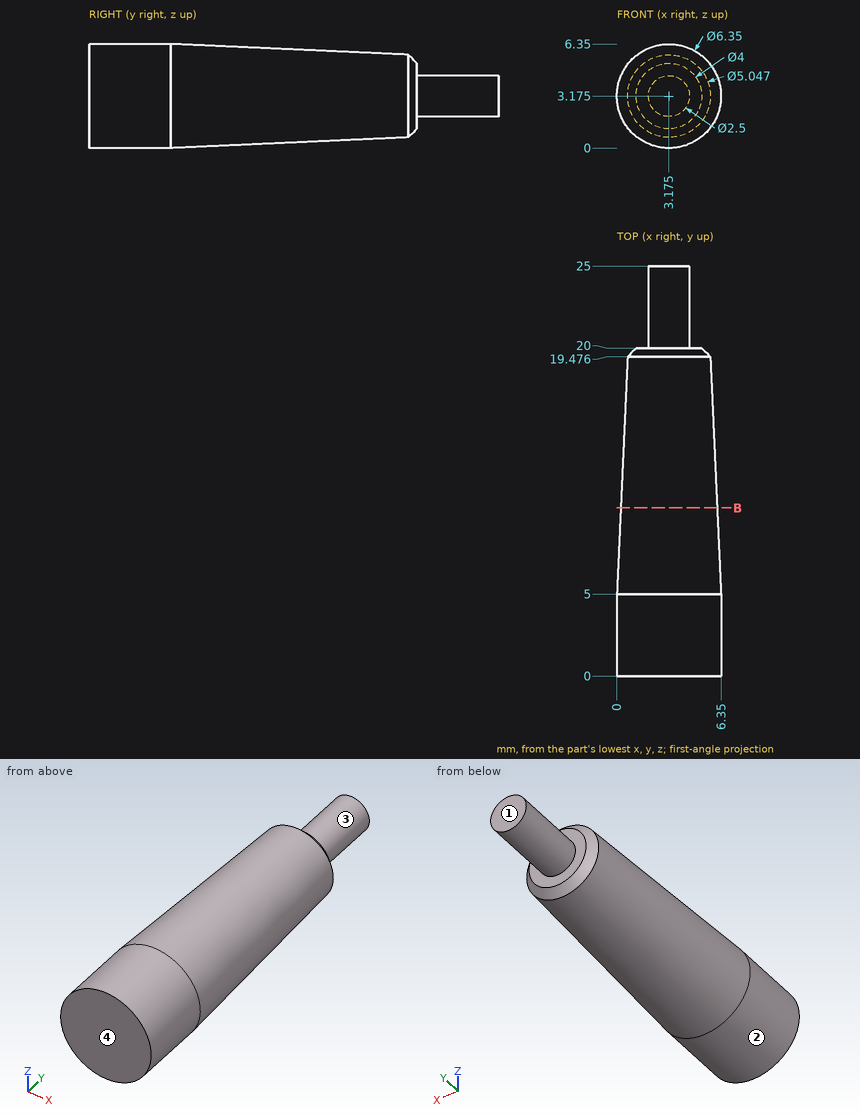
Source: three-view drawing plus pictorial views. Frame: mm from the lowest corner of the part. A direction names the side the tool comes from. Round coordinates to 2 decimals unless told otherwise and drop trailing zeros. Loops run counter-clockwise (first coordinate to the right, second up) from the corner with the lowest first, then second, coordinate; pieces in that order, holes last. Notation, with made-up numbers: M -27.75,-18.5 L 20.25,-18.5 A17 cw 20.25,-0.5 Z; hole C 43,39.25 d1. An arc over 180 degrees is marked long. Answer as CSV lines item,"result". Start each with the question number.
(1) Line query: line 1 (Y direction, x = 2.25, z = 1.5); line 2 (Z direction, x = 2, y = 6.75); line 3 (Z direction, x = 2.5, y = 16.75) (1 decimal). Output: solid intervals per line, ascending. Write a range as [from, to].
(2) First-contact query: pin 1 (3 mm diameter, centred on y = 4, z = 4.5, fed in from -X); pin 2 (2 mm diameter, centred on y = 14, z = 2.5, fed in from +X). Flat tips, straight axial feed; report the tip coordinate or a pass-through.
(3) Draft query along X for the marked faces 1 and 2. Return one class per face: released by +X, released by -X, zero draft, split by the parting line, or undercut.
(4) Section B-B, the plane y = 10.25. Output: boundary loops of the cut face in (x, z) (1 decimal), plus the area to 3 significant figures.
(5) Reachability of the marked faces 3 and 4 from +Z, -Z, +X, -X, +Y, -Y: full face, straight path, thin tool, end or side. Return the list, or none.
Values found:
1,line 1,"y = [0, 20]"
1,line 2,"z = [0.31, 6.04]"
1,line 3,"z = [0.6, 5.7]"
2,pin 1,"stops at x = 0"
2,pin 2,"stops at x = 5.98"
3,face 1,"zero draft"
3,face 2,"split by the parting line"
4,outline,"C 3.2,3.2 d5.9"
4,area,"27.1 mm²"
5,face 3,"+Y"
5,face 4,"+Z, -Z, +X, -X, -Y"
